```python
from build123d import *

# Parameters (mm, degrees)
SKETCH1_W           = 70
SKETCH1_H           = 10
BOSS_EXTRUDE1_DEPTH = 2
SKETCH2_R           = 1.5
CUT_EXTRUDE1_DEPTH  = 2
SKETCH3_R           = 1.5
CUT_EXTRUDE2_DEPTH  = 10


with BuildPart() as part:
    # Sketch1 → Boss-Extrude1 (new body)
    with BuildSketch(Plane.XY):
        with Locations((-35, -5)):
            Rectangle(SKETCH1_W, SKETCH1_H)
    extrude(amount=BOSS_EXTRUDE1_DEPTH)

    # Sketch2 → Cut-Extrude1 (cut)
    with BuildSketch(Plane.XY.offset(2)):
        with Locations((-5.07364211, -4.928592782)):
            Circle(SKETCH2_R)
    extrude(amount=-CUT_EXTRUDE1_DEPTH, mode=Mode.SUBTRACT)

    # Sketch3 → Cut-Extrude2 (cut)
    with BuildSketch(Plane.XY.offset(2)):
        with Locations((-50, -4.733233439)):
            Circle(SKETCH3_R)
    extrude(amount=-CUT_EXTRUDE2_DEPTH, mode=Mode.SUBTRACT)


solid = part.part
```
Could you check a few things on this model? Use its own coordinates, in mm. Round coordinates to 2 decimals unless told otherwise and drop trailing zeros. Loops run counter-clockwise (first coordinate to the right, second up) from the corner with the lowest first, then second, coordinate; pieces in that order, holes last. Notation, with made-up numbers: M -40,-8.75 L -24,-8.75 A20 cw -24,5.25 Z; hole C -8,67.25 d3. An arc over 180 degrees is marked long. Answer as CSV lines item,"result".
1) If I drill on probe 1 along X at (y, z) = (-4.25, 0.5); probe 2 along Y at (x, z) = (-50, 1.65); probe 3 along X at (y, z) = (-4.5, 0.45), over which ranges is the centre line in solid material (lowest first)?
From the geometry:
probe 1,"-70 to -51.42, -48.58 to -6.41, -3.74 to 0"
probe 2,"-10 to -6.23, -3.23 to 0"
probe 3,"-70 to -51.48, -48.52 to -6.51, -3.64 to 0"
2) Imagine slicing it at B-B on z = 1.65. List the corners of the cut face in (x, y) for me, and give its area (3 significant figures).
From the geometry:
outline,"M -70,-10 L 0,-10 L 0,0 L -70,0 Z; hole C -50,-4.73 d3; hole C -5.07,-4.93 d3"
area,"686 mm^2"
3) We'd pull the mould along X, two halves only. Please class faces 1 (the flat face through (-35, 0, 1)), 2 (the flat face through (-70, -5, 1)), 3 (the cylindrical face through (-6.179, -3.915, 1.014)): released by +X, released by -X, zero draft, split by the parting line, or undercut.
From the geometry:
face 1,"zero draft"
face 2,"released by -X"
face 3,"undercut"
4) For pin 1 Ø6 at (x, y) = (-29.5, -2.5) entering from -Z; pin 2 Ø2.5 at (x, y) = (-5.07, -4.93) entering from +Z, each with a flat end and sliding along its axis, tell me the tip position at first contact or that it passes through.
From the geometry:
pin 1,"z = 0"
pin 2,"through"
5) Imagine slicing it at A-A on x = -50. List the corners of the cut face in (y, z) for me, and give its area (3 significant figures).
From the geometry:
outline,"M -10,0 L -6.23,0 L -6.23,2 L -10,2 Z; M -3.23,0 L 0,0 L 0,2 L -3.23,2 Z"
area,"14.0 mm^2"
